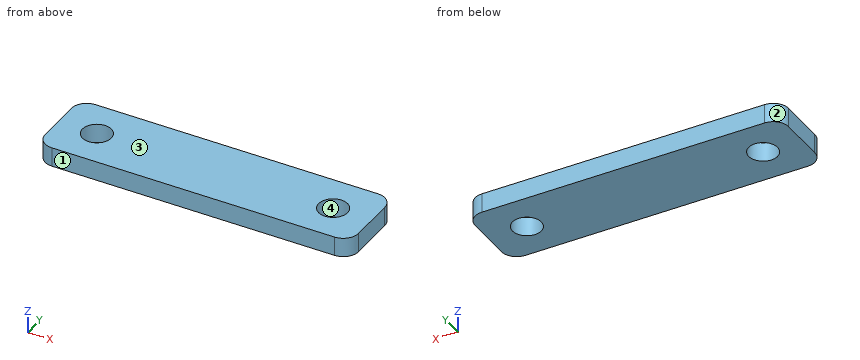
from build123d import *

# Parameters (mm, degrees)
SKETCH1_W           = 103.1875
SKETCH1_H           = 25.4
BOSS_EXTRUDE1_DEPTH = 6.35
FILLET1_R           = 5.08
SKETCH2_R           = 4.7625
CUT_EXTRUDE1_DEPTH  = 107.457233931


with BuildPart() as part:
    # Sketch1 → Boss-Extrude1 (new body)
    with BuildSketch(Plane.XY):
        with Locations((51.59375, 12.7)):
            Rectangle(SKETCH1_W, SKETCH1_H)
    extrude(amount=-BOSS_EXTRUDE1_DEPTH)

    # Fillet1
    fillet1_edges = [part.edges().sort_by_distance(p)[0] for p in [
        (0, 25.4, -3.175),
        (103.1875, 25.4, -3.175),
        (103.1875, 0, -3.175),
        (0, 0, -3.175),
    ]]
    fillet(fillet1_edges, radius=FILLET1_R)

    # Sketch2 → Cut-Extrude1 (cut, through all)
    with BuildSketch(Plane.XY):
        with Locations((12.7, 12.7)):
            Circle(SKETCH2_R)
        with Locations((90.4875, 12.7)):
            Circle(SKETCH2_R)
    extrude(amount=-CUT_EXTRUDE1_DEPTH, mode=Mode.SUBTRACT)


solid = part.part
Input: part model. Units: mm. Frame: model coordinates. Face numbers are marked on the shaded views. Give positions to 0.01 mm unless a question says otherwise; leave off trailing zeros. Write each loop counter-clockwise with the first axis right and the second up, starting at its lowest first coordinate (ties: lowest second). Pieces come first, ordered by that corner, then holes. Notation, with made-up numbers: (16, -35) -> (59, -35) arc R17 cw to (59, -19) -> close; hole circle Ø11 at (13, 25.25). An arc over 180 degrees is marked (long way). Use one line per item in the form item = value. Start each with the question number.
1) Section query A-A on y = 12.7. Count the separate pieces of the cut face and the enclosed holes in it, then the cut area to 3 significant figures.
2) Pin query (flat end, axial travel): pin 1 (8.5 mm diameter, centred on x = 12.7, y = 12.7, fed in from -Z). Return the tip coordinate at first contact, or that it passes through.
3) Section query B-B on x = 12.7. Return the cut outline in (y, z).
4) Section query D-D on x = 92. Return the cut outline in (y, z), then the cut area to 3 significant figures.
5) Draft query along Y for the marked faces 1, 2, 3 and 4. Return one class per face: pulls with the +Y half, pulls with the -Y half, needs draft (parallel to the pull), parting line crosses it, or undercut.
6) Ray query, probe 1 along Y at (x, z) = (12.7, -2.5); probe 2 along Y at (x, z) = (92, -1.5); probe 3 along X at (y, z) = (24, -5). Return the intervals inside material, ascending. Write a range as from..to.
Outcome:
q1.separate_pieces = 3
q1.enclosed_holes = 0
q1.area = 534 mm^2
q2.pin_1 = through
q3.outline = (0, -6.35) -> (7.94, -6.35) -> (7.94, 0) -> (0, 0) -> close; (17.46, -6.35) -> (25.4, -6.35) -> (25.4, 0) -> (17.46, 0) -> close
q4.outline = (0, -6.35) -> (8.18, -6.35) -> (8.18, 0) -> (0, 0) -> close; (17.22, -6.35) -> (25.4, -6.35) -> (25.4, 0) -> (17.22, 0) -> close
q4.area = 104 mm^2
q5.face_1 = pulls with the -Y half
q5.face_2 = pulls with the +Y half
q5.face_3 = needs draft
q5.face_4 = undercut
q6.probe_1 = 0..7.94, 17.46..25.4
q6.probe_2 = 0..8.18, 17.22..25.4
q6.probe_3 = 1.58..101.61
